from build123d import *

# Parameters (mm, degrees)
SKETCH1_R           = 2.5
BOSS_EXTRUDE2_DEPTH = 2.1
SKETCH10_W          = 5
SKETCH10_H          = 6
BOSS_EXTRUDE5_DEPTH = 2.5
SKETCH12_R          = 1
CUT_EXTRUDE1_DEPTH  = 2


with BuildPart() as part:
    # Sketch1 → Boss-Extrude2 (new body)
    with BuildSketch(Plane(origin=(0, 0, 0), x_dir=(1, 0, 0), z_dir=(0, 1, 0))):
        with Locations(Location((0, 0, 0), (0, 0, 270))):
            Circle(SKETCH1_R)
    extrude(amount=BOSS_EXTRUDE2_DEPTH)

    # Sketch10 → Boss-Extrude5 (add)
    with BuildSketch(Plane(origin=(2.5, 0, 0), x_dir=(0, 0, -1), z_dir=(1, 0, 0))):
        with Locations((0, 3)):
            Rectangle(SKETCH10_W, SKETCH10_H)
    extrude(amount=-BOSS_EXTRUDE5_DEPTH)

    # Sketch11 → Cut-Revolve2 (revolve, cut)
    with BuildSketch(Plane.ZY):
        with BuildLine():
            Line((-1.386997153, 4), (1.613002847, 4))
            ThreePointArc((1.613002847, 4), (0.113002847, 5.5), (-1.386997153, 4))
        make_face()
    revolve(axis=Axis((0, 4, -1.386997153), (0, 0, 1)), mode=Mode.SUBTRACT)

    # Sketch12 → Cut-Extrude1 (cut)
    with BuildSketch(Plane.XZ):
        with Locations(Location((0, 0, 0), (0, 0, 270))):
            Circle(SKETCH12_R)
    extrude(amount=-CUT_EXTRUDE1_DEPTH, mode=Mode.SUBTRACT)


solid = part.part
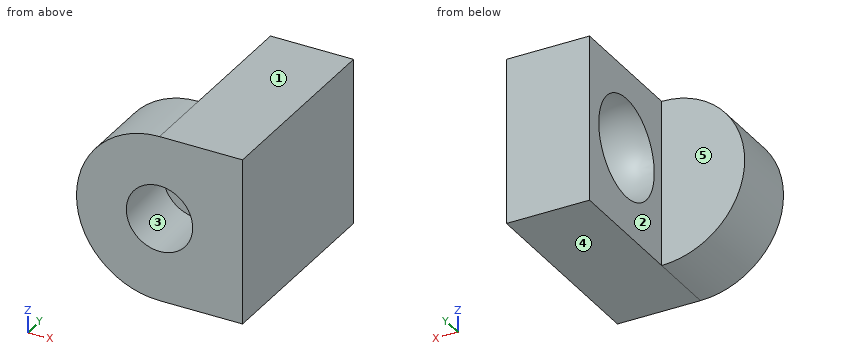
Source: CAD feature listing. Evaluate the final solid. Frame: model axes, mm. Face numbers are marked on the shaded views. A direction names the side the tool comes from. Coordinates: 2 decimals unless noted, no trailing zeros. Order: outer loops, then holes, each group sorted by start corner. A loop starts at its lowest first (then second) coordinate and runs counter-clockwise, first axis right, second up. Notation, with made-up numbers: M 45.5,4.5 L 53.5,4.5 A17 ccw 53.5,31.5 Z; hole C 87,44 d10. An arc over 180 degrees is marked long. Write each question's results on one line, items separated by ' | '. Start each with the question number.
Item 1: Cut plane A-A (z = -1.15). Return loops of the section in (x, y), and give its area (3 significant figures).
Item 2: Set-up query: the marked faces 1 and 2. Return all of +Z, -Z, +X, -X, +Y, -Y with unobstructed straight access to the full face (end or side cutting, diameter ignored); none if empty.
Item 3: Line query: probe 1 along X at (y, z) = (2.35, -1.9); probe 2 along Y at (x, z) = (-1.65, 0.2); probe 3 along Y at (x, z) = (0.6, 1.05). Output: solid intervals per line, ascending.
Item 4: Cut plane D-D (x = 1.2). Return loops of the section in (y, z), and give its area (3 significant figures).
Item 5: Cut plane B-B (x = -0.45). Return loops of the section in (y, z).
Item 6: Cut plane C-C (y = 3.65). Return loops of the section in (x, z).
Item 7: First-contact query: pin 1 Ø1 at (x, z) = (-1, -2) entering from +Y; pin 2 Ø1 at (x, y) = (-1.5, 3) entering from +Z. Flat tips, straight axial feed; report the tip coordinate or a pass-through.
Item 8: Draft query along Z for the marked faces 3, 4 and 5. Return one class per face: pulls with the +Z half, pulls with the -Z half, needs draft (parallel to the pull), parting line crosses it, or undercut.
Checked values:
1) outline: M -2.22,0 L 2.5,0 L 2.5,6 L 0,6 L 0,4.81 A0.81 cw 0,3.19 L 0,2.1 L -2.22,2.1 Z | area: 18.6 mm2
2) face 1: +Z, +X, -X, +Y, -Y | face 2: +Z, -Z, -X, +Y
3) probe 1: x = 0 to 2.5 | probe 2: y = 0 to 2.1 | probe 3: y = 0 to 2.99, 5.01 to 6
4) outline: M 0,-2.5 L 6,-2.5 L 6,2.5 L 0,2.5 Z; hole C 4,0.11 d1.8 | area: 27.5 mm2
5) outline: M 0,-2.46 L 2.1,-2.46 L 2.1,2.46 L 0,2.46 L 0,0.89 L 2,0.89 L 2,-0.89 L 0,-0.89 Z
6) outline: M 0,-2.5 L 2.5,-2.5 L 2.5,2.5 L 0,2.5 L 0,1.57 A1.46 cw 0,-1.35 Z
7) pin 1: stops at y = 2.1 | pin 2: passes through
8) face 3: undercut | face 4: pulls with the -Z half | face 5: needs draft
